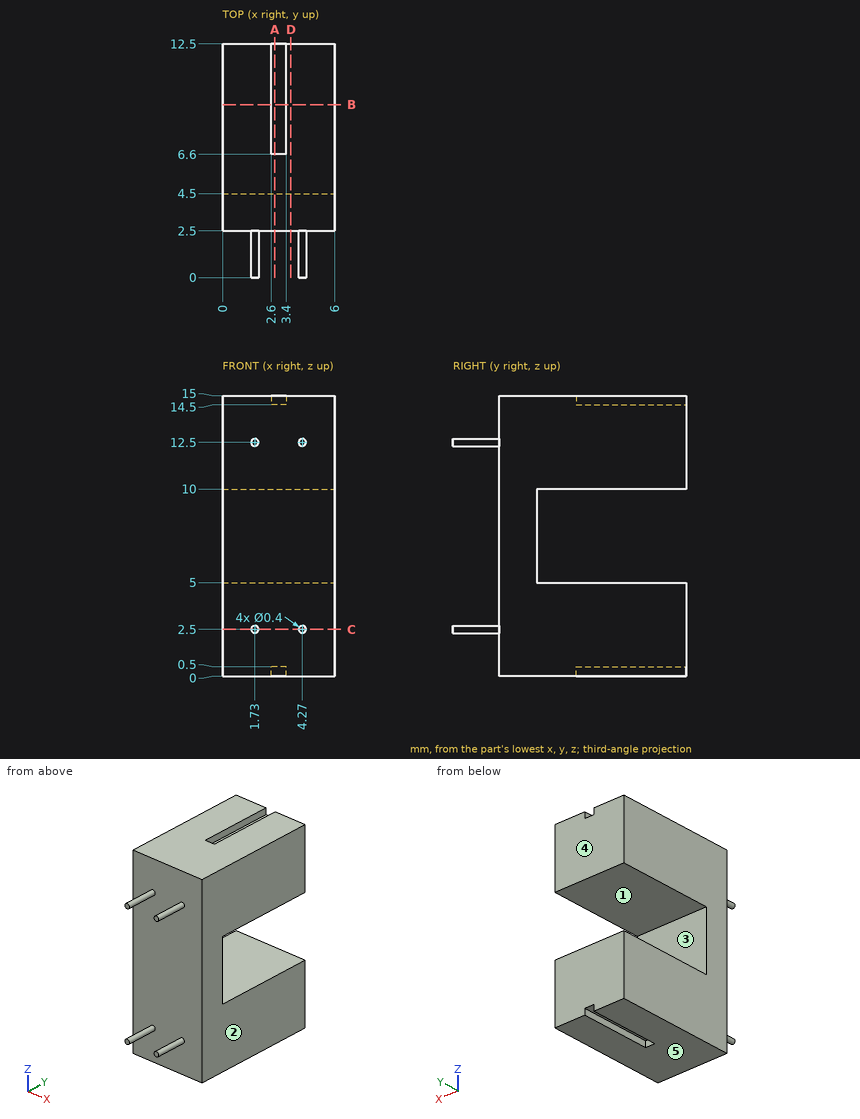
Could you check a few things on this drawing? It's one solid part, dimensions in mm from its lowest x, y, z. A direction names the side the tool comes from. Round coordinates to 2 decimals unless told otherwise and drop trailing zeros. Write each loop counter-clockwise with the first axis right and the second up, starting at its lowest first coordinate (ties: lowest second). Pieces come first, ordered by that corner, then holes.
Q1. If we section it at A-A on x = 2.8: Write out the boundary of the cut face in (y, z).
Q2. If we section it at B-B on y = 9.25: Write out the boundary of the cut face in (x, z).
Q3. If we mould it in two halves opening along Z, with no side actions, what happens to the marked faces 3, 4 and 5? For each: +Z half, -Z half, draft (parallel to the pull), parting line (faces both ways), or undercut.
Q4. If we section it at C-C on z = 2.5: Write out the boundary of the cut face in (x, y).
Q5. If we section it at D-D on x = 3.65: Write out the boundary of the cut face in (y, z).
Q6. Will these pins go through, and if not, where does the flat tip stop? P1, Ø2.5, axis at x = 3, z = 8, coming from the +Y side; P2, Ø1.5, axis at x = 4, z = 9, coming from the -Y side.
Q7. Please list where these lines run through material, in increasing order: probe 1 along Z at (x, y) = (5.75, 6.25); probe 2 along Z at (x, y) = (4.3, 2); probe 3 along Y at (x, z) = (1, 4.75).
Q8. Which directions (+Z, -Z, +X, -X, +Y, -Y) give clear straight access to the entire face, cutting with the end or side of a thin tool? Please do the marked faces 1 and 2.
Answer below:
1. outline: (2.5, 0) - (6.6, 0) - (6.6, 0.5) - (12.5, 0.5) - (12.5, 5) - (4.5, 5) - (4.5, 10) - (12.5, 10) - (12.5, 14.5) - (6.6, 14.5) - (6.6, 15) - (2.5, 15) - close
2. outline: (0, 0) - (2.6, 0) - (2.6, 0.5) - (3.4, 0.5) - (3.4, 0) - (6, 0) - (6, 5) - (0, 5) - close; (0, 10) - (6, 10) - (6, 15) - (3.4, 15) - (3.4, 14.5) - (2.6, 14.5) - (2.6, 15) - (0, 15) - close
3. face 3: undercut
3. face 4: draft
3. face 5: -Z half
4. outline: (0, 2.5) - (1.53, 2.5) - (1.53, 0) - (1.93, 0) - (1.93, 2.5) - (4.07, 2.5) - (4.07, 0) - (4.47, 0) - (4.47, 2.5) - (6, 2.5) - (6, 12.5) - (0, 12.5) - close
5. outline: (2.5, 0) - (12.5, 0) - (12.5, 5) - (4.5, 5) - (4.5, 10) - (12.5, 10) - (12.5, 15) - (2.5, 15) - close
6. P1: stops at y = 4.5
6. P2: stops at y = 2.5
7. probe 1: z = 0 to 5, 10 to 15
7. probe 2: z = 2.3 to 2.7, 12.3 to 12.7
7. probe 3: y = 2.5 to 12.5
8. face 1: +X, -X, +Y
8. face 2: +Z, -Z, +X, +Y, -Y
